from build123d import *

# Parameters (mm, degrees)
SZKIC1_W                   = 4.7
SZKIC1_H                   = 4.08
WYTNIJ_WYCI_GNI_CIE1_DEPTH = 6.6
ZAOKR_GLENIE1_R            = 0.6


with BuildPart() as part:
    # Szkic1 → Obrót1 (revolve)
    with BuildSketch(Plane(origin=(0, 0, 0), x_dir=(1, 0, 0), z_dir=(0, 1, 0)), mode=Mode.PRIVATE) as obr_t1_sk:
        Polygon((0, -33.5), (0, -22.5), (-8, -22.5), (-12, -22.5), (-12, -33.5), align=None)
        Polygon((0, -22.5), (0, 22.5), (-4.7, 22.5), (-8, 22.5), (-8, -22.5), align=None)
        with Locations((-2.35, 24.54)):
            Rectangle(SZKIC1_W, SZKIC1_H)
        Polygon((-4.7, 26.58), (0, 26.58), (0, 40.5), (-4.7, 40.5), (-6, 39.3), (-6, 28.6), align=None)
    revolve(obr_t1_sk.sketch.rotate(Axis((0, 0, 33.5), (0, 0, -1)), 180), axis=Axis((0, 0, 33.5), (0, 0, -1)))

    # Szkic2 → Wytnij-wyciągnięcie1 (cut)
    with BuildSketch(Plane.XY.offset(33.5)):
        Polygon((4, 2.309401077), (0, 4.618802154), (-4, 2.309401077), (-4, -2.309401077), (0, -4.618802154), (4, -2.309401077), align=None)
    extrude(amount=-WYTNIJ_WYCI_GNI_CIE1_DEPTH, mode=Mode.SUBTRACT)

    # Zaokrąglenie1
    zaokr_glenie1_edges = [part.edges().sort_by_distance(p)[0] for p in [
        (-12, 0, 33.5),
    ]]
    fillet(zaokr_glenie1_edges, radius=ZAOKR_GLENIE1_R)


solid = part.part
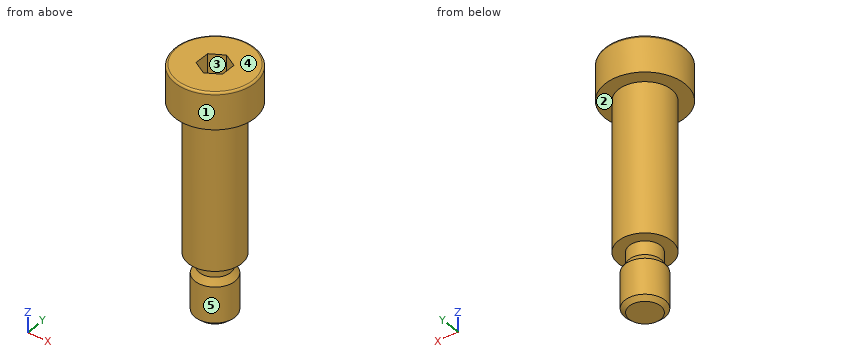
The model under review builds one solid part; all positions refer to its coordinate system, in mm. Face numbers are marked on the shaded views. A direction names the side the tool comes from. Round coordinates to 2 decimals unless told otherwise and drop trailing zeros. Write each loop counter-clockwise with the first axis right and the second up, starting at its lowest first coordinate (ties: lowest second). Pieces come first, ordered by that corner, then holes. Notation, with made-up numbers: (74.25, -19) -> (86.25, -19) arc R12 cw to (86.25, -4) -> close; hole circle Ø9 at (82.5, -7). An arc over 180 degrees is marked (long way). Answer as a JSON object with one key per item and string values.
1. Machinability: for the marked faces 4 and 5, which of the approach directions +Z, -Z, +X, -X, +Y, -Y give a long, thin tool a straight path to every point of the face, cutting with its end or side? Answer none if there is none.
Results found:
{"face 4": "+Z, +X, -X, +Y, -Y", "face 5": "-Z"}
2. We need section C-C on z = 17.5. State the section outline as (x, y) points, and give its area (3 significant figures).
Results found:
{"outline": "circle Ø16 at (0, 0)", "area": "201 mm^2"}
3. To check wall thickness, follow line 1 along Z through (x, y) = (8.25, -1.75); line 2 along X through (y, z) = (-0.25, -11.5); line 3 along Z through (x, y) = (-4.25, -3.75). State the ranges of each line that lie inside material, in increasing order.
Results found:
{"line 1": "z = 22.5 to 33.5", "line 2": "x = -8 to 8", "line 3": "z = -39.61 to -28.08, -22.5 to 33.5"}
4. The part is to be moulded in two halves that separate along X. For the marked faces 1, 2 and 3, say which applies: pulls with the +X half, pulls with the -X half, needs draft (parallel to the pull), parting line crosses it, or undercut.
Results found:
{"face 1": "parting line crosses it", "face 2": "needs draft", "face 3": "undercut"}
5. We need section A-A on y = 0. State the section outline as (x, z) points.
Results found:
{"outline": "(-12, 22.5) -> (-8, 22.5) -> (-8, -22.5) -> (-4.7, -22.5) -> (-4.7, -26.58) -> (-6, -28.6) -> (-6, -39.3) -> (-4.7, -40.5) -> (4.7, -40.5) -> (6, -39.3) -> (6, -28.6) -> (4.7, -26.58) -> (4.7, -22.5) -> (8, -22.5) -> (8, 22.5) -> (12, 22.5) -> (12, 32.9) arc R0.6 ccw to (11.4, 33.5) -> (4, 33.5) -> (4, 26.9) -> (-4, 26.9) -> (-4, 33.5) -> (-11.4, 33.5) arc R0.6 ccw to (-12, 32.9) -> close"}
6. We need section B-B on z = -31. State the section outline as (x, y) points, and give its area (3 significant figures).
Results found:
{"outline": "circle Ø12 at (0, 0)", "area": "113 mm^2"}
7. Clearance check with flat-ended pins moving along their axes: pin 1 (12 mm diameter, centred on x = -3.5, y = -4.5, fed in from -Z); pin 2 (3 mm diameter, centred on x = -0.5, z = -4.5, fed in from +Y); pin 3 (1.4 mm diameter, centred on y = 1, z = 31.5, fed in from +X); pin 4 (8 mm diameter, centred on y = 7, z = 20, fed in from +X). State where each tip first meets the part, or that it passes through.
Results found:
{"pin 1": "stops at z = -40.5", "pin 2": "stops at y = 8", "pin 3": "stops at x = 12", "pin 4": "stops at x = 11.36"}
